Build history of the part. All positions in model axes, mm. Face numbers are marked on the shaded views. A direction names the side the tool comes from. Round coordinates to 2 decimals unless told otherwise and drop trailing zeros. Write each loop counter-clockwise with the first axis right and the second up, starting at its lowest first coordinate (ties: lowest second). Pieces come first, ordered by that corner, then holes. Notation, with made-up numbers: (25.25, -17) - (42.25, -17) arc R23 cw to (42.25, -9) - close; hole circle Ø8 at (2, 7). An arc over 180 degrees is marked (long way). Answer as a JSON object with one key per item and string values. Group by question number.
Item 1: Which spindle directions (+Z, -Z, +X, -X, +Y, -Y) get a long thin tool onto all of the face, cutting with end or side? Do the marked faces 1, 2 and 3. Say none if no direction does.
Item 2: Two-plate mould, pull along X, no slides. Class the marked faces 4, 5, 6 and 7: +X half, -X half, draft (parallel to the pull), parting line (faces both ways), or undercut.
Item 3: Flat gauge pins, fed straight in: pin 1 (2 mm diameter, centred on x = 7, z = 9, fed in from +Y); pin 2 (3.5 mm diameter, centred on y = 43, z = 32, fed in from -X); pin 3 (1.5 mm diameter, centred on x = 6.5, y = 5.5, fed in from +Z). Where does each tip first touch, or does it go through?
Item 4: Slice it at A-A, the plane y = 23. List the corners of the cut face in (x, z), then the cut area to 3 significant figures.
Item 5: Slice it at C-C, the plane z = 6.5. List the corners of the cut face in (x, y), then the cut area to 3 significant figures.
Item 6: Slice it at B-B, the plane x = -10.5. List the corners of the cut face in (y, z), then the cut area to 3 significant figures.
Item 7: Probe line 1 (Z direction, x = 0, y = 25.5); line 2 (X direction, y = 11.5, z = 26); line 3 (Y direction, x = 17, z = -3). List the from-to ranges inside material, lowest first. Write a range as from..to.
Item 8: Slice it at D-D, the plane x = 4. List the corners of the cut face in (y, z).
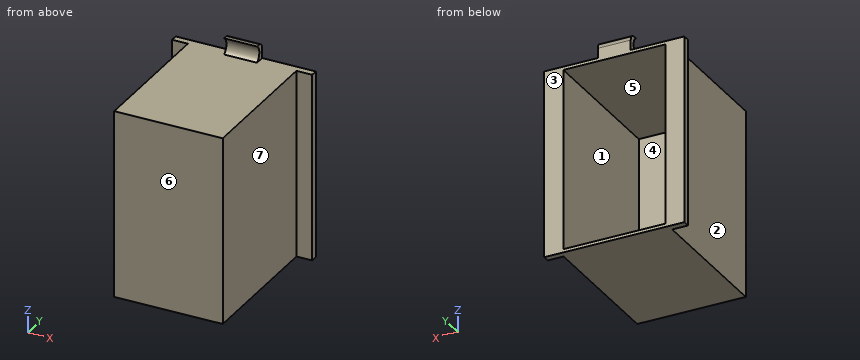
from build123d import *

# Parameters (mm, degrees)
SKETCH1_W           = 33
SKETCH1_H           = 57
BOSS_EXTRUDE1_DEPTH = 45
SHELL1_T            = -1
SKETCH3_W           = 57
SKETCH3_H           = 2.1
BOSS_EXTRUDE2_DEPTH = 4.8
SKETCH4_W           = 10
SKETCH4_H           = 3
BOSS_EXTRUDE3_DEPTH = 5
CUT_EXTRUDE1_DEPTH  = 10
FILLET2_R           = 2


with BuildPart() as part:
    # Sketch1 → Boss-Extrude1 (new body)
    with BuildSketch(Plane(origin=(0, 0, 0), x_dir=(1, 0, 0), z_dir=(0, 1, 0))):
        Rectangle(SKETCH1_W, SKETCH1_H)
    extrude(amount=BOSS_EXTRUDE1_DEPTH)

    # Shell1
    shell1_openings = [part.faces().sort_by_distance(p)[0] for p in [
        (0, 45, 0),
    ]]
    offset(amount=SHELL1_T, openings=shell1_openings, kind=Kind.INTERSECTION)

    # Sketch3 → Boss-Extrude2 (add)
    with BuildSketch(Plane.ZY.offset(16.5)):
        with Locations((0, 43.95)):
            Rectangle(SKETCH3_W, SKETCH3_H)
    boss_extrude2 = extrude(amount=BOSS_EXTRUDE2_DEPTH)

    # Mirror1: Boss-Extrude2 across plane
    add(boss_extrude2.mirror(Plane(origin=(0, 0, 0), x_dir=(0, 0, 1), z_dir=(1, 0, 0))))

    # Sketch4 → Boss-Extrude3 (add)
    with BuildSketch(Plane.XY.offset(28.5)):
        with Locations((0, 43.5)):
            Rectangle(SKETCH4_W, SKETCH4_H)
    extrude(amount=BOSS_EXTRUDE3_DEPTH)

    # Sketch5 → Cut-Extrude1 (cut)
    with BuildSketch(Plane.ZY.offset(5)):
        with BuildLine():
            Line((28.5, 42), (33.5, 42))
            ThreePointArc((33.5, 42), (31, 43.341687605), (28.5, 42))
        make_face()
    extrude(amount=-CUT_EXTRUDE1_DEPTH, mode=Mode.SUBTRACT)

    # Fillet2
    fillet2_edges = [part.edges().sort_by_distance(p)[0] for p in [
        (0, 45, 33.5),
    ]]
    fillet(fillet2_edges, radius=FILLET2_R)


solid = part.part
Geometry says:
{
 "1": {"face 1": "+Y", "face 2": "+Z, -Z, -X, -Y", "face 3": "+Z, -Z, +X, -X, +Y"},
 "2": {"face 4": "undercut", "face 5": "undercut", "face 6": "draft", "face 7": "+X half"},
 "3": {"pin 1": "stops at y = 1", "pin 2": "stops at x = -5", "pin 3": "stops at z = 28.5"},
 "4": {"outline": "(-16.5, -28.5) - (16.5, -28.5) - (16.5, 28.5) - (-16.5, 28.5) - close; hole (-15.5, -27.5) - (15.5, -27.5) - (15.5, 27.5) - (-15.5, 27.5) - close", "area": "176 mm^2"},
 "5": {"outline": "(-21.3, 42.9) - (-16.5, 42.9) - (-16.5, 0) - (16.5, 0) - (16.5, 42.9) - (21.3, 42.9) - (21.3, 45) - (15.5, 45) - (15.5, 1) - (-15.5, 1) - (-15.5, 45) - (-21.3, 45) - close", "area": "141 mm^2"},
 "6": {"outline": "(0, -28.5) - (45, -28.5) - (45, -27.5) - (1, -27.5) - (1, 27.5) - (45, 27.5) - (45, 28.5) - (0, 28.5) - close", "area": "145 mm^2"},
 "7": {"line 1": "z = -28.5..-27.5, 27.5..28.5", "line 2": "x = -16.5..-15.5, 15.5..16.5", "line 3": "y = 42.9..45"},
 "8": {"outline": "(0, -28.5) - (45, -28.5) - (45, -27.5) - (1, -27.5) - (1, 27.5) - (45, 27.5) - (45, 31.5) arc R2 ccw to (43, 33.5) - (42, 33.5) arc R3 cw to (42, 28.5) - (0, 28.5) - close"}
}
